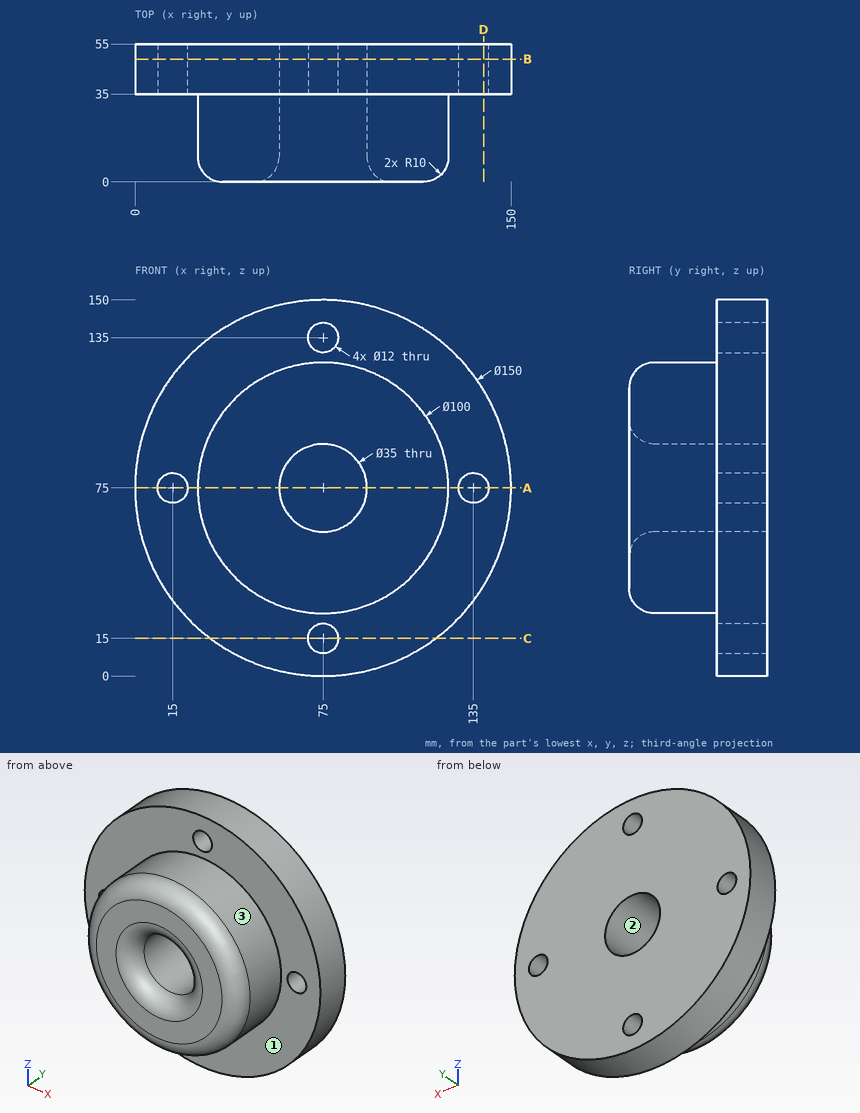
Design review of the part shown in the three views and the two pictorial views. Dimensions are in mm from the part's minimum x, y and z. Give positions to 0.01 mm unless a question says otherwise; leave off trailing zeros. Loops run counter-clockwise (first coordinate to the right, second up) from the corner with the lowest first, then second, coordinate; pieces in that order, holes last. Notation, with made-up numbers: M 3,76.5 L 10,76.5 A25 cw 10,92.5 Z; hole C 19,76.5 d3. An arc over 180 degrees is marked long. Answer as a JSON object with one key per item and string values. Group by question number.
Q1. Mouldability with a two-part tool opening along X and no side actions: class the marked faces 1, 2 and 3 as +X half, -X half, draft (parallel to the pull), parting line (faces both ways), or undercut.
Q2. Insertion check: P1, Ø4, axis at x = 59.5, y = 7.5, coming from the +Z side; P2, Ø11, axis at x = 75, z = 135, coming from the -Y side; P3, Ø3, axis at y = 14, z = 74.5, coming from the -X side; P4, Ø15.5, axis at x = 75, z = 15, coming from the -Y side. Each pin has a flat end and moves straight along its axis. Give the tip position at first contact, or say it passes through.
Q3. Add section A-A on z = 75. Give the boundary of the cut face in (x, y).
Q4. Add section D-D on x = 139. Give the boundary of the cut face in (y, z), and give its area (3 significant figures).
Q5. For probe 1 along Z at (x, y) = (75, 45); probe 2 along X at (y, z) = (33, 75); probe 3 along Y at (x, z) = (7, 58.5), list the stretches that pass through material, from the lowest coordinate up. Write a range as [from, to].
Q6. Add section C-C on z = 15. Give the boundary of the cut face in (x, y).
Q7. Add section B-B on y = 49. Give the boundary of the cut face in (x, z), and give its area (3 significant figures).
Checked values:
{
 "1": {"face 1": "draft", "face 2": "undercut", "face 3": "parting line"},
 "2": {"P1": "z = 122.95", "P2": "through", "P3": "x = 25", "P4": "y = 35"},
 "3": {"outline": "M 0,35 L 9,35 L 9,55 L 0,55 Z; M 21,35 L 25,35 L 25,10 A10 ccw 35,0 L 47.5,0 A10 ccw 57.5,10 L 57.5,55 L 21,55 Z; M 92.5,10 A10 ccw 102.5,0 L 115,0 A10 ccw 125,10 L 125,35 L 129,35 L 129,55 L 92.5,55 Z; M 141,35 L 150,35 L 150,55 L 141,55 Z"},
 "4": {"outline": "M 35,35.9 L 55,35.9 L 55,70.53 L 35,70.53 Z; M 35,79.47 L 55,79.47 L 55,114.1 L 35,114.1 Z", "area": "1,390 mm²"},
 "5": {"probe 1": "[0, 9], [21, 57.5], [92.5, 129], [141, 150]", "probe 2": "[25, 57.5], [92.5, 125]", "probe 3": "[35, 55]"},
 "6": {"outline": "M 30,35 L 69,35 L 69,55 L 30,55 Z; M 81,35 L 120,35 L 120,55 L 81,55 Z"},
 "7": {"outline": "C 75,75 d150; hole C 15,75 d12; hole C 75,75 d35; hole C 75,15 d12; hole C 75,135 d12; hole C 135,75 d12", "area": "16,300 mm²"}
}
